CAD build for the part. Positions are in the model's coordinates, mm. A direction names the side the tool comes from. Round coordinates to 2 decimals unless told otherwise and drop trailing zeros. Loops run counter-clockwise (first coordinate to the right, second up) from the corner with the lowest first, then second, coordinate; pieces in that order, holes last. Notation, with made-up numbers: (14, 57.25) - (65, 57.25) arc R27 cw to (65, 93.25) - close; hole circle Ø4 at (36.5, 81). An arc over 180 degrees is marked (long way). Use one line per item in the form item = value.
from build123d import *

# Parameters (mm, degrees)
CYLINDER082_R             = 2
CYLINDER082_DEPTH         = 28
CYLINDER083_R             = 3.75
CYLINDER083_DEPTH         = 2
CYLINDER084_R             = 3.75
CYLINDER084_DEPTH         = 1
CYLINDER085_R             = 3
CYLINDER085_DEPTH         = 8
CYLINDER086_R             = 4
CYLINDER086_DEPTH         = 6
CYLINDER087_R             = 1
CYLINDER087_DEPTH         = 2
FUSION026_PLACEMENT_ANGLE = 180


with BuildPart() as cylinder082:
    # Cylinder082 → Cylinder082 (new body)
    with BuildSketch(Plane.XY):
        Circle(CYLINDER082_R)
    extrude(amount=CYLINDER082_DEPTH)


with BuildPart() as cylinder083:
    # Cylinder083 → Cylinder083 (new body)
    with BuildSketch(Plane.XY.offset(5)):
        Circle(CYLINDER083_R)
    extrude(amount=CYLINDER083_DEPTH)


with BuildPart() as cylinder084:
    # Cylinder084 → Cylinder084 (new body)
    with BuildSketch(Plane.XY.offset(11)):
        Circle(CYLINDER084_R)
    extrude(amount=CYLINDER084_DEPTH)


with BuildPart() as cylinder085:
    # Cylinder085 → Cylinder085 (new body)
    with BuildSketch(Plane.XY.offset(12)):
        Circle(CYLINDER085_R)
    extrude(amount=CYLINDER085_DEPTH)


with BuildPart() as cylinder086:
    # Cylinder086 → Cylinder086 (new body)
    with BuildSketch(Plane.XY.offset(20)):
        Circle(CYLINDER086_R)
    extrude(amount=CYLINDER086_DEPTH)


with BuildPart() as fusion025:
    # Cone001 → Cone001 (revolve)
    with BuildSketch(Plane(origin=(0, 0, 26), x_dir=(1, 0, 0), z_dir=(0, -1, 0))):
        Polygon((0, 0), (4, 0), (3.5, 2), (0, 2), align=None)
    revolve(axis=Axis((0, 0, 26), (0, 0, 1)))

    # Fusion025: union Cylinder082, Cylinder083, Cylinder084, Cylinder085, Cylinder086
    add(cylinder082.part)
    add(cylinder083.part)
    add(cylinder084.part)
    add(cylinder085.part)
    add(cylinder086.part)


with BuildPart() as obj1:
    # Cylinder087 → Cylinder087 (new body)
    with BuildSketch(Plane.XY.offset(-2)):
        Circle(CYLINDER087_R)
    extrude(amount=CYLINDER087_DEPTH)

    # Fusion026: union Fusion025
    add(fusion025.part)


with BuildPart() as obj1_1:
    # Fusion026 placement: moved
    add(obj1.part.moved(Location((0, -289, -301.5))).rotate(Axis((0, -289, -301.5), (0, -1, 0)), FUSION026_PLACEMENT_ANGLE))


solid = obj1_1.part
1) Drill centre lines: probe 1 along Z at (x, y) = (3, -289.5); probe 2 along Z at (x, y) = (-1, -287); probe 3 along Z at (x, y) = (-0.25, -290). Where is each one in solid material? Low to high.
Report:
probe_1 = -329.5 to -321.5, -313.5 to -312.5, -308.5 to -306.5
probe_2 = -329.5 to -312.5, -308.5 to -306.5
probe_3 = -329.5 to -301.5
2) Slice it at C-C (z = -305.5). Write the cut outline in (x, y), plus the area to 3 significant figures.
Report:
outline = circle Ø4 at (0, -289)
area = 12.6 mm^2
3) Flat gauge pins, fed straight in: pin 1 (4 mm diameter, centred on x = -2.5, z = -309, fed in from +Y); pin 2 (1 mm diameter, centred on x = 0.5, z = -313, fed in from -Y); pin 3 (4 mm diameter, centred on y = -290, z = -311.5, fed in from -X). Where does each tip first touch, or does it go through?
Report:
pin_1 = -285.29
pin_2 = -292.75
pin_3 = -3.75
4) Tool access for faces 1 (the cylindrical face through (0, -288, -300)), 2 (the cylindrical face through (-1.846, -292.549, -324.458)), 3 (the flat face through (-2, -291, -308.5)): list every direction of +Z, -Z, +X, -X, +Y, -Y with a clear straight run to the whole face (end or side of a thin tool).
Report:
face_1 = +Z
face_2 = +Z, -Z
face_3 = none
5) Two-plate mould, pull along Z, no slides. Class faces 4 (the flat face through (0, -289, -329.5)), 5 (the flat face through (-2, -291, -306.5)), 6 (the flat face through (-1, -286, -313.5)): +Z half, -Z half, draft (parallel to the pull), parting line (faces both ways), or undercut.
Report:
face_4 = -Z half
face_5 = +Z half
face_6 = undercut
